Here's how the part is built. I have some questions about the finished solid (model axes, mm). Face numbers are marked on the shaded views. A direction names the side the tool comes from. Round coordinates to 2 decimals unless told otherwise and drop trailing zeros. Write each loop counter-clockwise with the first axis right and the second up, starting at its lowest first coordinate (ties: lowest second). Pieces come first, ordered by that corner, then holes. Notation, with made-up numbers: M -39,75 L -16,75 A27 ccw -16,95 Z; hole C 73,9.5 d10. An arc over 180 degrees is marked long. Write item = value, one per line. Start each with the question number.
(1) On a 3-axis mill with a long thin cutter (end or side, diameter ignored), from which of +Z, -Z, +X, -X, +Y, -Y can I reach the whole of each face in a straight line? I mean the marked faces 1 and 2. Say none if no direction works.
(2) Will these pins go through, and if not, where does the flat tip stop? pin 1 Ø2 at (x, z) = (5, 6) entering from +Y; pin 2 Ø10 at (x, y) = (12.5, 66) entering from +Z; pin 3 Ø2 at (y, z) = (57.5, 10) entering from +X.
(3) I want a section at C-C (x = 12). List the corners of the cut face in (y, z) for me, and give its area (3 significant figures).
(4) I need wall thicknesses on line 1 along Z through (x, y) = (10.5, 53). Which ranges of the line are inside material? Lowest first, please.
(5) I want a section at B-B (y = 85.5). List the corners of the cut face in (x, z) for me, and give its area (3 significant figures).
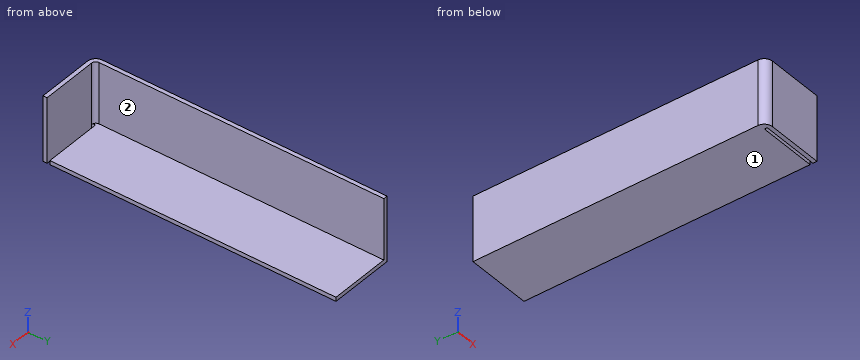
Autodesk Inventor part; units mm, degrees
ref_plane "YZ Plane" through (0, 0, 0) normal (1, 0, 0) x (0, 1, 0)
ref_plane "XZ Plane" through (0, 0, 0) normal (0, 1, 0) x (-1, 0, 0)
ref_plane "XY Plane" through (0, 0, 0) normal (0, 0, 1) x (1, 0, 0)
sketch "Sketch1" plane through (0, 0, 0) normal (0, 0, 1) x (1, 0, 0)
  line L0 (0, 0) -> (25.4, 0)
  line L1 (25.4, 114.3) -> (0, 114.3)
  line L2 (0, 114.3) -> (0, 0)
  line L3 (25.4, 1.5875) -> (1.5875, 1.5875)
  line L4 (1.5875, 1.5875) -> (1.5875, 114.3)
  line L5 (25.4, 2.6988) -> (3.175, 2.6987)
  arc A0 (3.175, 2.6987) -> (3.175, 1.5875) centre (3.175, 2.1431) ccw
  line L6 (25.4, 0) -> (25.4, 1.5875)
  line L7 (25.4, 2.6988) -> (25.4, 114.3)
  dimension "d0" = 25.4
  dimension "d1" = 114.3
  dimension "d2" = 1.5875
  dimension "d3" = 1.5875
  dimension "d4" = 1.1113
  dimension "d5" = 1.5875
extrude "Extrusion1" add sketch "Sketch1" along normal blind 25.4 contours L2 L1 L4 L3 L6 L0
extrude "Extrusion2" add sketch "Sketch1" along normal blind 1.5875 contours L1 L7 L5 A0 L3 L4
fillet "Fillet1" radius 1.5875 1 edges at (1.5875, 1.5875, 13.4938)
fillet "Fillet2" radius 3.175 1 edges at (0, 0, 12.7)
equation "\"d2\" = d3"
equation "\"d4\" = 0.7 * d2"
properties part number "dozer side mid mount"
Returned:
q1.face_1 = -Z, +X, -X, +Y, -Y
q1.face_2 = +Z, +X, +Y
q2.pin_1 = 1.59
q2.pin_2 = 1.59
q2.pin_3 = 1.59
q3.outline = M 0,0 L 1.59,0 L 1.59,25.4 L 0,25.4 Z; M 2.7,0 L 114.3,0 L 114.3,1.59 L 2.7,1.59 Z
q3.area = 217 mm²
q4.line_1 = 0 to 1.59
q5.outline = M 0,0 L 25.4,0 L 25.4,1.59 L 1.59,1.59 L 1.59,25.4 L 0,25.4 Z
q5.area = 78.1 mm²
